Design review of the part built by this model. Coordinates are the model's own, in mm. A direction names the side the tool comes from. Round coordinates to 2 decimals unless told otherwise and drop trailing zeros. Order: outer loops, then holes, each group sorted by start corner. A loop starts at its lowest first (then second) coordinate and runs counter-clockwise, first axis right, second up. Notation, with made-up numbers: (24.25, 76) - (75.25, 76) arc R14 ccw to (75.25, 82) - close; hole circle Ø7 at (-13.5, -4). An arc over 180 degrees is marked (long way). Use CSV: the item, a comma, the result in double quotes.
from build123d import *

# Parameters (mm, degrees)
SKETCH1_R           = 50.8
BOSS_EXTRUDE1_DEPTH = 248.79
SKETCH3_R           = 16.256
CUT_EXTRUDE1_DEPTH  = 25.4
SKETCH4_R           = 2.413
CUT_EXTRUDE2_DEPTH  = 102.6000001
SKETCH5_R           = 3.935994996
SKETCH5_R_2         = 5.186201194
BOSS_EXTRUDE2_DEPTH = 3.81


with BuildPart() as part:
    # Sketch1 → Boss-Extrude1 (new body)
    with BuildSketch(Plane(origin=(0, 0, 0), x_dir=(1, 0, 0), z_dir=(0, 1, 0))):
        Circle(SKETCH1_R)
    extrude(amount=BOSS_EXTRUDE1_DEPTH)

    # Sketch3 → Cut-Extrude1 (cut)
    with BuildSketch(Plane.XY.offset(50.8)):
        with Locations((0, 147.668)):
            Circle(SKETCH3_R)
    extrude(amount=-CUT_EXTRUDE1_DEPTH, mode=Mode.SUBTRACT)

    # Sketch4 → Cut-Extrude2 (cut, through all)
    with BuildSketch(Plane(origin=(50.8, 0, 0), x_dir=(0, 0, -1), z_dir=(1, 0, 0))):
        with Locations((0, 186.79)):
            Circle(SKETCH4_R)
        with Locations((0, 94.58)):
            Circle(SKETCH4_R)
        with Locations((0, 25.4)):
            Circle(SKETCH4_R)
    extrude(amount=-CUT_EXTRUDE2_DEPTH, mode=Mode.SUBTRACT)

    # Sketch5 → Boss-Extrude2 (add)
    with BuildSketch(Plane(origin=(0, 248.79, 0), x_dir=(1, 0, 0), z_dir=(0, 1, 0))):
        with Locations((0, 41.48960955)):
            Circle(SKETCH5_R)
        with Locations((0, -36.918720362)):
            Circle(SKETCH5_R_2)
    extrude(amount=BOSS_EXTRUDE2_DEPTH)


solid = part.part
1) We need section D-D (y = 25.4). Give the boundary of the cut face in (x, z), then the cut area to 3 significant figures.
Data:
outline,"(-50.74, -2.41) arc R50.8 ccw to (50.74, -2.41) - close; (-50.74, 2.41) - (50.74, 2.41) arc R50.8 ccw to start"
area,"7,620 mm2"
2) Insertion check: pin 1 Ø8 at (x, z) = (16.5, -40.5) entering from +Y; pin 2 Ø1 at (x, z) = (0.5, -37) entering from -Y; pin 3 Ø5 at (y, z) = (191.5, -32) entering from -X; pin 4 Ø2 at (y, z) = (44, 8) entering from -X. Each pin has a flat end and moves straight along its axis. Give the tip position at first contact, or say it passes through.
Data:
pin 1,"stops at y = 248.79"
pin 2,"stops at y = 0"
pin 3,"stops at x = -41.36"
pin 4,"stops at x = -50.32"
3) We need section C-C (z = 28). Give the boundary of the cut face in (x, y), then the cut area to 3 significant figures.
Data:
outline,"(-42.39, 0) - (42.39, 0) - (42.39, 248.79) - (-42.39, 248.79) - close; hole circle Ø32.51 at (0, 147.67)"
area,"20,300 mm2"
4) We need section A-A (x = 0). Give the boundary of the cut face in (y, z).
Data:
outline,"(0, -50.8) - (248.79, -50.8) - (248.79, -45.43) - (252.6, -45.43) - (252.6, -37.55) - (248.79, -37.55) - (248.79, 31.73) - (252.6, 31.73) - (252.6, 42.1) - (248.79, 42.1) - (248.79, 50.8) - (163.92, 50.8) - (163.92, 25.4) - (131.41, 25.4) - (131.41, 50.8) - (0, 50.8) - close; hole circle Ø4.83 at (25.4, 0); hole circle Ø4.83 at (94.58, 0); hole circle Ø4.83 at (186.79, 0)"
5) We need section B-B (z = 0). Give the boundary of the cut face in (x, y).
Data:
outline,"(-50.8, 0) - (50.8, 0) - (50.8, 22.99) - (-50.8, 22.99) - close; (-50.8, 27.81) - (50.8, 27.81) - (50.8, 92.17) - (-50.8, 92.17) - close; (-50.8, 96.99) - (50.8, 96.99) - (50.8, 184.38) - (-50.8, 184.38) - close; (-50.8, 189.2) - (50.8, 189.2) - (50.8, 248.79) - (-50.8, 248.79) - close"
6) The part is to be moulded in two halves that separate along Y. For faces 1 (the face through (-0.853, 250.668, -37.647)), 2 (the face through (0.711, 23.044, 0.523)), 3 (the face through (-1, 0, -1)), say which applies: +Y half, -Y half, draft (parallel to the pull), parting line (faces both ways), or undercut.
Data:
face 1,"draft"
face 2,"undercut"
face 3,"-Y half"
7) For faces 4 (the face through (2.39, 250.67, 41.52)), 5 (the face through (0, 148, 25.4)), 6 (the face through (0, 252.6, -42)), list the 3-axis set-ups (+Z, -Z, +X, -X, +Y, -Y) from which the entire face can be reached by the end or side of a thin tool; tool diameter is ignored.
Data:
face 4,"+Y"
face 5,"+Z"
face 6,"+Z, -Z, +X, -X, +Y"
8) To check wall thickness, follow L1, parallel to Y at x = -28.5, z = 0; L2, parallel to Y at x = 31, z = 26.5; L3, parallel to X at y = 82, z = 2. State the ranges of each line that lie inside material, in increasing order. Write a range as from..to.
Data:
L1,"y = 0..22.99, 27.81..92.17, 96.99..184.38, 189.2..248.79"
L2,"y = 0..248.79"
L3,"x = -50.76..50.76"
